```python
from build123d import *

# Parameters (mm, degrees)
SKETCH2_R           = 20
BOSS_EXTRUDE2_DEPTH = 5
SKETCH3_W           = 5
SKETCH3_H           = 5
BOSS_EXTRUDE3_DEPTH = 43
SKETCH4_R           = 2.5
BOSS_EXTRUDE4_DEPTH = 41
SKETCH5_W           = 7.704684196
SKETCH5_H           = 10
CUT_EXTRUDE1_DEPTH  = 6
FILLET1_R           = 2
CHAMFER1_SIZE       = 1


with BuildPart() as part:
    # Sketch2 → Boss-Extrude2 (new body)
    with BuildSketch(Plane(origin=(0, 0, 0), x_dir=(0, 0, -1), z_dir=(1, 0, 0))):
        Circle(SKETCH2_R)
    extrude(amount=BOSS_EXTRUDE2_DEPTH)

    # Sketch3 → Boss-Extrude3 (add)
    with BuildSketch(Plane(origin=(5, 0, 0), x_dir=(0, 0, -1), z_dir=(1, 0, 0))):
        Rectangle(SKETCH3_W, SKETCH3_H)
    extrude(amount=BOSS_EXTRUDE3_DEPTH)

    # Sketch4 → Boss-Extrude4 (add)
    with BuildSketch(Plane(origin=(5, 0, 0), x_dir=(0, 0, -1), z_dir=(1, 0, 0))):
        with Locations((-8.485281374, 8.485281374)):
            Circle(SKETCH4_R)
        with Locations((8.485281374, -8.485281374)):
            Circle(SKETCH4_R)
    extrude(amount=BOSS_EXTRUDE4_DEPTH)

    # Sketch5 → Cut-Extrude1 (cut, through all)
    with BuildSketch(Plane(origin=(5, 0, 0), x_dir=(0, 0, -1), z_dir=(1, 0, 0))):
        with BuildLine():
            Line((-12, 16), (-3.852342098, 16))
            Line((-3.852342098, 16), (-3.852342098, 19.625479876))
            ThreePointArc((-3.852342098, 19.625479876), (-8.130818752, 18.272651324), (-12, 16))
        make_face()
        with BuildLine():
            Line((-3.852342098, 19.625479876), (-3.852342098, 16))
            Line((-3.852342098, 16), (3.852342098, 16))
            Line((3.852342098, 16), (3.852342098, 19.625479876))
            ThreePointArc((3.852342098, 19.625479876), (1.935252254, 19.906149771), (2.3e-08, 20))
            ThreePointArc((2.3e-08, 20), (-1.935252231, 19.906149773), (-3.852342098, 19.625479876))
        make_face()
        with BuildLine():
            Line((3.852342098, 19.625479876), (3.852342098, 16))
            Line((3.852342098, 16), (12, 16))
            ThreePointArc((12, 16), (8.130818752, 18.272651324), (3.852342098, 19.625479876))
        make_face()
        with Locations((0, 11)):
            Rectangle(SKETCH5_W, SKETCH5_H)
    extrude(amount=-CUT_EXTRUDE1_DEPTH, mode=Mode.SUBTRACT)

    # Fillet1
    fillet1_edges = [part.edges().sort_by_distance(p)[0] for p in [
        (2.5, 16, 12),
        (2.5, 16, -12),
        (2.5, 16, -3.852342098),
        (2.5, 16, 3.852342098),
    ]]
    fillet(fillet1_edges, radius=FILLET1_R)

    # Chamfer1
    chamfer1_edges = [part.edges().sort_by_distance(p)[0] for p in [
        (5, 8.485281374, 10.985281374),
        (5, -8.485281374, -5.985281374),
    ]]
    chamfer(chamfer1_edges, length=CHAMFER1_SIZE)


solid = part.part
```
Build history of the part. All positions in model axes, mm. A direction names the side the tool comes from. Round coordinates to 2 decimals unless told otherwise and drop trailing zeros. Order: outer loops, then holes, each group sorted by start corner. A loop starts at its lowest first (then second) coordinate and runs counter-clockwise, first axis right, second up. Notation, with made-up numbers: (81, 62) -> (101, 62) arc R28 ccw to (101, 83) -> close; hole circle Ø11 at (-2.5, 50.5). An arc over 180 degrees is marked (long way). Answer in a Markdown table with one row per item.
1) Which spindle directions (+Z, -Z, +X, -X, +Y, -Y) get a long thin tool onto all of the face, cutting with end or side? Do faces 1 (the flat face through (26, 0, -2.5)), 2 (the cylindrical face through (2.465, 15.399, 4.423)), 3 (the flat face through (26, 0, 2.5)), 4 (the flat face through (26, 2.5, 0)). Say none if no direction does.
Values:
| item | result |
|---|---|
| face 1 | -Z, +X, +Y, -Y |
| face 2 | +X, -X, +Y |
| face 3 | +Z, +X, +Y, -Y |
| face 4 | +Z, -Z, +X, +Y |
2) Band-saw the part on C-C on x = 29. Give the cut face in (y, z), and give its area (3 significant figures).
Values:
| item | result |
|---|---|
| outline | circle Ø5 at (-8.49, -8.49); (-2.5, -2.5) -> (2.5, -2.5) -> (2.5, 2.5) -> (-2.5, 2.5) -> close; circle Ø5 at (8.49, 8.49) |
| area | 64.3 mm2 |
3) Band-saw the part on A-A on z = 0. Give the cut face in (x, y).
Values:
| item | result |
|---|---|
| outline | (0, -20) -> (5, -20) -> (5, -2.5) -> (48, -2.5) -> (48, 2.5) -> (5, 2.5) -> (5, 6) -> (0, 6) -> close |
4) Wall check: L1, parallel to Y at x = 35, z = 1; L2, parallel to X at y = -11, z = 12. Give the ranges that are in metal, low to high.
Values:
| item | result |
|---|---|
| L1 | -2.5 to 2.5 |
| L2 | 0 to 5 |
5) Band-saw the part on D-D on z = -17. Give the cut face in (x, y), and give its area (3 significant figures).
Values:
| item | result |
|---|---|
| outline | (0, -10.54) -> (5, -10.54) -> (5, 10.54) -> (0, 10.54) -> close |
| area | 105 mm2 |
6) Band-saw the part on B-B on y = 0. Give the cut face in (x, z), and give its area (3 significant figures).
Values:
| item | result |
|---|---|
| outline | (0, -20) -> (5, -20) -> (5, -2.5) -> (48, -2.5) -> (48, 2.5) -> (5, 2.5) -> (5, 20) -> (0, 20) -> close |
| area | 415 mm2 |
7) Mould opens along Z. For faces 5 (the cylindrical face through (2.465, 15.43, -4.454)), 6 (the cylindrical face through (2.465, 15.882, -11.989)), 7 (the cylindrical face through (25.72, 6.964, 10.469)), 8 (the flat face through (26, -2.5, 0)) say: released by +Z, released by -Z, zero draft, split by the parting line, or undercut.
Values:
| item | result |
|---|---|
| face 5 | undercut |
| face 6 | released by -Z |
| face 7 | split by the parting line |
| face 8 | zero draft |
8) Pin check, flat tips, straight feed: P1, Ø1.5, axis at x = 36, y = 9.5, coming from the +Z side; P2, Ø1.5, axis at x = 33.5, y = 0.5, coming from the -Z side; P3, Ø12, axis at x = 33.5, z = -12.5, coming from the +Y side. Stop position of each tip, or through.
Values:
| item | result |
|---|---|
| P1 | z = 10.97 |
| P2 | z = -2.5 |
| P3 | y = -5.99 |
